The model under review builds one solid part; all positions refer to its coordinate system, in mm. Round coordinates to 2 decimals unless told otherwise and drop trailing zeros. Loops run counter-clockwise (first coordinate to the right, second up) from the corner with the lowest first, then second, coordinate; pieces in that order, holes last. Notation, with made-up numbers: (68, 73.25) -> (123, 73.25) arc R13 ccw to (123, 81.25) -> close; hole circle Ø8 at (86, 17). An arc over 180 degrees is marked (long way). Write each question's results on one line, items separated by ' | '. Start each with the question number.
Item 1: Mouldability with a two-part tool opening along Y and no side actions: class faces 1 (the flat face through (2.9, 0, 1)), 2 (the flat face through (0, 0, 2.38)) as pulls with the +Y half, pulls with the -Y half, needs draft (parallel to the pull), parting line crosses it, or undercut.
Item 2: We need section C-C (z = 0.85). Give the boundary of the cut face in (x, y), and give its area (3 significant figures).
Item 3: We need section D-D (y = 1.75). Give the boundary of the cut face in (x, z), and give its area (3 significant figures).
Item 4: We need section B-B (x = 2.75). Give the boundary of the cut face in (y, z), and give its area (3 significant figures).
Item 5: For L1, parallel to X at y = 3, z = 2.15; L2, parallel to Y at x = -1.25, z = 1.8, list the stretches that pass through material, from the lowest coordinate up. Write a range as from..to.
Item 6: Clearance check with flat-ended pins moving along their axes: pin 1 Ø0.6 at (x, y) = (2.5, 2) entering from -Z; pin 2 Ø1 at (y, z) = (-0.5, 1) entering from +X; pin 3 Ø0.7 at (x, z) = (-0.5, 1) entering from -Y. State where each tip first meets the part, or that it passes through.
Item 7: We need section A-A (y = 0). Give the boundary of the cut face in (x, z), and give its area (3 significant figures).
from build123d import *

# Parameters (mm, degrees)
SKETCH1_W           = 6.2
SKETCH1_H           = 6.2
BOSS_EXTRUDE1_DEPTH = 2.38
SKETCH2_W           = 2
SKETCH2_H           = 0.8
CUT_EXTRUDE1_DEPTH  = 0.4
SKETCH3_W           = 6.2
SKETCH3_H           = 0.1
CUT_EXTRUDE2_DEPTH  = 7.2
SKETCH14_W          = 0.2
SKETCH14_H          = 3.2
CUT_EXTRUDE3_DEPTH  = 2
SKETCH16_W          = 2
SKETCH16_H          = 0.2
CUT_EXTRUDE4_DEPTH  = 7.2
SKETCH19_W          = 0.61
SKETCH19_H          = 0.2
CUT_EXTRUDE5_DEPTH  = 1.28
SKETCH20_W          = 0.2
SKETCH20_H          = 0.8
CUT_EXTRUDE6_DEPTH  = 0.6
FILLET1_R           = 0.05


with BuildPart() as part:
    # Sketch1 → Boss-Extrude1 (new body)
    with BuildSketch(Plane.XY):
        Rectangle(SKETCH1_W, SKETCH1_H)
    extrude(amount=BOSS_EXTRUDE1_DEPTH)

    # Sketch2 → Cut-Extrude1 (cut)
    with BuildSketch(Plane(origin=(0, 0, 0), x_dir=(-1, 0, 0), z_dir=(0, 0, -1))):
        with Locations((-2.1, 2)):
            Rectangle(SKETCH2_W, SKETCH2_H)
        with Locations((2.1, 2)):
            Rectangle(SKETCH2_W, SKETCH2_H)
        with Locations((2.1, -2)):
            Rectangle(SKETCH2_W, SKETCH2_H)
        with Locations((-2.1, -2)):
            Rectangle(SKETCH2_W, SKETCH2_H)
    extrude(amount=-CUT_EXTRUDE1_DEPTH, mode=Mode.SUBTRACT)

    # Sketch3 → Cut-Extrude2 (cut, through all)
    with BuildSketch(Plane(origin=(0, 3.1, 0), x_dir=(1, 0, 0), z_dir=(0, 1, 0))):
        with Locations((0, -0.05)):
            Rectangle(SKETCH3_W, SKETCH3_H)
    extrude(amount=-CUT_EXTRUDE2_DEPTH, mode=Mode.SUBTRACT)

    # Sketch14 → Cut-Extrude3 (cut)
    with BuildSketch(Plane(origin=(0, 0, 0.1), x_dir=(-1, 0, 0), z_dir=(0, 0, -1))):
        with Locations((3, 0)):
            Rectangle(SKETCH14_W, SKETCH14_H)
        with Locations((-3, 0)):
            Rectangle(SKETCH14_W, SKETCH14_H)
    extrude(amount=-CUT_EXTRUDE3_DEPTH, mode=Mode.SUBTRACT)

    # Sketch16 → Cut-Extrude4 (cut, through all)
    with BuildSketch(Plane.ZY.offset(3.1)):
        with Locations((1.1, -3)):
            Rectangle(SKETCH16_W, SKETCH16_H)
        with Locations((1.1, 3)):
            Rectangle(SKETCH16_W, SKETCH16_H)
    extrude(amount=-CUT_EXTRUDE4_DEPTH, mode=Mode.SUBTRACT)

    # Sketch19 → Cut-Extrude5 (cut, through all)
    with BuildSketch(Plane(origin=(0, 0, 2.1), x_dir=(-1, 0, 0), z_dir=(0, 0, -1))):
        with Locations((-2.605, -3)):
            Rectangle(SKETCH19_W, SKETCH19_H)
        with Locations((2.605, -3)):
            Rectangle(SKETCH19_W, SKETCH19_H)
        with Locations((2.605, 3)):
            Rectangle(SKETCH19_W, SKETCH19_H)
        with Locations((-2.605, 3)):
            Rectangle(SKETCH19_W, SKETCH19_H)
    extrude(amount=-CUT_EXTRUDE5_DEPTH, mode=Mode.SUBTRACT)

    # Sketch20 → Cut-Extrude6 (cut)
    with BuildSketch(Plane(origin=(0, 0, 0.4), x_dir=(-1, 0, 0), z_dir=(0, 0, -1))):
        with Locations((-3, -2)):
            Rectangle(SKETCH20_W, SKETCH20_H)
        with Locations((-3, 2)):
            Rectangle(SKETCH20_W, SKETCH20_H)
        with Locations((3, 2)):
            Rectangle(SKETCH20_W, SKETCH20_H)
        with Locations((3, -2)):
            Rectangle(SKETCH20_W, SKETCH20_H)
    extrude(amount=-CUT_EXTRUDE6_DEPTH, mode=Mode.SUBTRACT)

    # Fillet1
    fillet1_edges = [part.edges().sort_by_distance(p)[0] for p in [
        (2.3, -3.1, 2.24),
        (0, -3.1, 2.1),
        (-2.3, -3.1, 2.24),
        (0, -3.1, 2.38),
        (-2.3, 3.1, 2.24),
        (0, 3.1, 2.1),
        (2.3, 3.1, 2.24),
        (0, 3.1, 2.38),
        (-3.1, -1.6, 1.55),
        (-3.1, 0, 2.1),
        (-3.1, 1.6, 1.55),
        (-3.1, 2, 1),
        (-3.1, 2.4, 0.55),
        (-3.1, 2.9, 1.1),
        (-3.1, 3, 2.1),
        (-3.1, 3.1, 2.24),
        (-3.1, 0, 2.38),
        (-3.1, -3.1, 2.24),
        (-3.1, -3, 2.1),
        (-3.1, -2.9, 1.1),
        (-3.1, -2.4, 0.55),
        (-3.1, -2, 1),
        (-2.1, 2.4, 0.1),
        (-1.1, 2, 0.1),
        (-2, 1.6, 0.1),
        (-2.9, 0, 0.1),
        (-2, -1.6, 0.1),
        (-1.1, -2, 0.1),
        (-2.1, -2.4, 0.1),
        (-3.1, -2.65, 0.1),
        (0, -2.9, 0.1),
        (2.1, -2.4, 0.1),
        (1.1, -2, 0.1),
        (2, -1.6, 0.1),
        (2.9, 0, 0.1),
        (2, 1.6, 0.1),
        (1.1, 2, 0.1),
        (2.1, 2.4, 0.1),
        (0, 2.9, 0.1),
        (-3.1, 2.65, 0.1),
        (3.1, 1.6, 1.55),
        (3.1, 0, 2.1),
        (3.1, -1.6, 1.55),
        (3.1, -2, 1),
        (3.1, -2.4, 0.55),
        (3.1, -2.65, 0.1),
        (3.1, -2.9, 1.1),
        (3.1, -3, 2.1),
        (3.1, -3.1, 2.24),
        (3.1, 0, 2.38),
        (3.1, 3.1, 2.24),
        (3.1, 3, 2.1),
        (3.1, 2.9, 1.1),
        (3.1, 2.65, 0.1),
        (3.1, 2.4, 0.55),
        (3.1, 2, 1),
        (3.005, -3.1, 2.1),
        (-2.91, -3.1, 2.24),
        (-2.91, -3, 2.1),
        (3.005, 3.1, 2.1),
        (2.91, 3.1, 2.24),
        (-3.005, 3.1, 2.1),
        (-2.91, 2.9, 2.24),
    ]]
    fillet(fillet1_edges, radius=FILLET1_R)


solid = part.part
Here are the results:
1) face 1: undercut | face 2: needs draft
2) outline: (-3.1, -2.85) arc R0.05 ccw to (-3.05, -2.9) -> (3.05, -2.9) arc R0.05 ccw to (3.1, -2.85) -> (3.1, -2.45) arc R0.05 ccw to (3.05, -2.4) -> (2.9, -2.4) -> (2.9, 2.4) -> (3.05, 2.4) arc R0.05 ccw to (3.1, 2.45) -> (3.1, 2.85) arc R0.05 ccw to (3.05, 2.9) -> (-3.05, 2.9) arc R0.05 ccw to (-3.1, 2.85) -> (-3.1, 2.45) arc R0.05 ccw to (-3.05, 2.4) -> (-2.9, 2.4) -> (-2.9, -2.4) -> (-3.05, -2.4) arc R0.05 ccw to (-3.1, -2.45) -> close | area: 34.0 mm2
3) outline: (-3.1, 1.05) arc R0.05 ccw to (-3.05, 1) -> (-2.9, 1) -> (-2.9, 0.4) -> (-1.1, 0.4) -> (-1.1, 0.15) arc R0.05 ccw to (-1.05, 0.1) -> (1.05, 0.1) arc R0.05 ccw to (1.1, 0.15) -> (1.1, 0.4) -> (2.9, 0.4) -> (2.9, 1) -> (3.05, 1) arc R0.05 ccw to (3.1, 1.05) -> (3.1, 2.33) arc R0.05 ccw to (3.05, 2.38) -> (-3.05, 2.38) arc R0.05 ccw to (-3.1, 2.33) -> close | area: 12.7 mm2
4) outline: (-2.9, 0.15) arc R0.05 ccw to (-2.85, 0.1) -> (-2.45, 0.1) arc R0.05 ccw to (-2.4, 0.15) -> (-2.4, 0.4) -> (-1.6, 0.4) -> (-1.6, 0.15) arc R0.05 ccw to (-1.55, 0.1) -> (1.55, 0.1) arc R0.05 ccw to (1.6, 0.15) -> (1.6, 0.4) -> (2.4, 0.4) -> (2.4, 0.15) arc R0.05 ccw to (2.45, 0.1) -> (2.85, 0.1) arc R0.05 ccw to (2.9, 0.15) -> (2.9, 2.38) -> (-2.9, 2.38) -> close | area: 12.7 mm2
5) L1: x = -3.1..-2.91, -2.3..2.3, 2.91..3.1 | L2: y = -2.9..2.9
6) pin 1: stops at z = 0.4 | pin 2: stops at x = 2.9 | pin 3: stops at y = -2.9
7) outline: (-3.1, 2.15) arc R0.05 ccw to (-3.05, 2.1) -> (-2.9, 2.1) -> (-2.9, 0.15) arc R0.05 ccw to (-2.85, 0.1) -> (2.85, 0.1) arc R0.05 ccw to (2.9, 0.15) -> (2.9, 2.1) -> (3.05, 2.1) arc R0.05 ccw to (3.1, 2.15) -> (3.1, 2.33) arc R0.05 ccw to (3.05, 2.38) -> (-3.05, 2.38) arc R0.05 ccw to (-3.1, 2.33) -> close | area: 13.3 mm2
